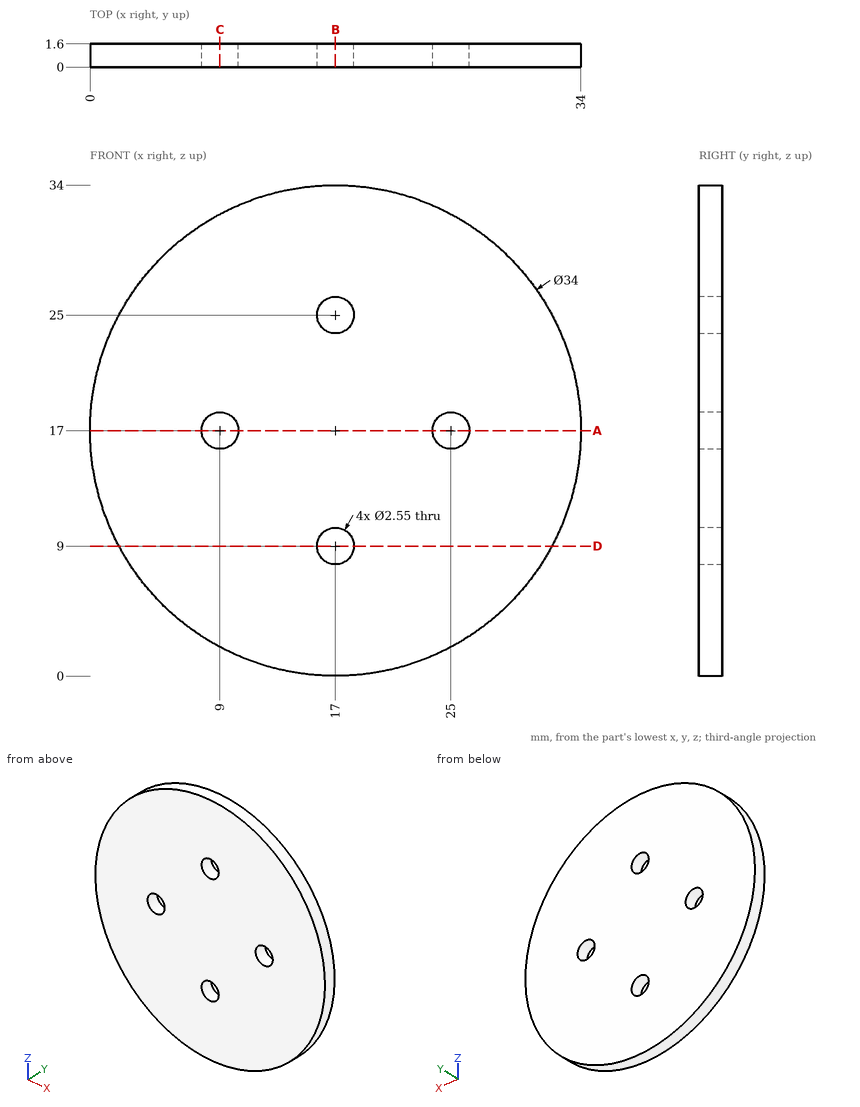
Job drawing, mm, ordinate dimensions from the low corner. One solid piece. Round coordinates to 2 decimals unless told otherwise and drop trailing zeros. Loops run counter-clockwise (first coordinate to the right, second up) from the corner with the lowest first, then second, coordinate; pieces in that order, holes last.
Item 1: Cut at C-C, the plane x = 9. Give the cut face in (y, z) (3 decimals).
Item 2: Cut at B-B, the plane x = 17. Give the cut face in (y, z) (3 decimals).
Item 3: Cut at A-A, the plane z = 17. Give the cut face in (x, y) (3 decimals), then the cut area to 3 significant figures.
Item 4: Drill centre lines: line 1 (X direction, y = 0.9, z = 17) (3 decimals); line 2 (X direction, y = 0.4, z = 9) (3 decimals); line 3 (Z direction, x = 8, y = 1.3). Where is each one in solid material? Low to high.
Item 5: Cut at D-D, the plane z = 9. Give the cut face in (x, y) (3 decimals).
A:
1. outline: (0, 2) - (1.6, 2) - (1.6, 15.725) - (0, 15.725) - close; (0, 18.275) - (1.6, 18.275) - (1.6, 32) - (0, 32) - close
2. outline: (0, 0) - (1.6, 0) - (1.6, 7.725) - (0, 7.725) - close; (0, 10.275) - (1.6, 10.275) - (1.6, 23.725) - (0, 23.725) - close; (0, 26.275) - (1.6, 26.275) - (1.6, 34) - (0, 34) - close
3. outline: (0, 0) - (7.725, 0) - (7.725, 1.6) - (0, 1.6) - close; (10.275, 0) - (23.725, 0) - (23.725, 1.6) - (10.275, 1.6) - close; (26.275, 0) - (34, 0) - (34, 1.6) - (26.275, 1.6) - close
3. area: 46.2 mm2
4. line 1: x = 0 to 7.725, 10.275 to 23.725, 26.275 to 34
4. line 2: x = 2 to 15.725, 18.275 to 32
4. line 3: z = 2.58 to 16.21, 17.79 to 31.42
5. outline: (2, 0) - (15.725, 0) - (15.725, 1.6) - (2, 1.6) - close; (18.275, 0) - (32, 0) - (32, 1.6) - (18.275, 1.6) - close
